Here's how the part is built. I have some questions about the finished solid (model axes, mm). Round coordinates to 2 decimals unless told otherwise and drop trailing zeros. Order: outer loops, then holes, each group sorted by start corner. A loop starts at its lowest first (then second) coordinate and runs counter-clockwise, first axis right, second up.
```python
from build123d import *

# Parameters (mm, degrees)
SKETCH1_W           = 20
SKETCH1_H           = 60
SKETCH1_R           = 3.3
BOSS_EXTRUDE1_DEPTH = 9.5
CHAMFER1_SIZE       = 0.3


with BuildPart() as part:
    # Sketch1 → Boss-Extrude1 (new body)
    with BuildSketch(Plane(origin=(0, 0, 0), x_dir=(1, 0, 0), z_dir=(0, 1, 0))):
        Rectangle(SKETCH1_W, SKETCH1_H)
        with Locations((0, 23)):
            Circle(SKETCH1_R, mode=Mode.SUBTRACT)
        with Locations((0, -23)):
            Circle(SKETCH1_R, mode=Mode.SUBTRACT)
    extrude(amount=BOSS_EXTRUDE1_DEPTH)

    # Chamfer1
    chamfer1_edges = [part.edges().sort_by_distance(p)[0] for p in [
        (-10, 4.75, -30),
        (10, 4.75, -30),
        (10, 4.75, 30),
        (-10, 4.75, 30),
    ]]
    chamfer(chamfer1_edges, length=CHAMFER1_SIZE)


solid = part.part
```
1. I need wall thicknesses on probe 1 along Z at (x, y) = (0, 4.5); probe 2 along X at (y, z) = (6.75, -23); probe 3 along Z at (x, y) = (-1.5, 3.5). Which ranges of each line are inside material? Lowest first, please.
Evaluation:
probe 1: z = -30 to -26.3, -19.7 to 19.7, 26.3 to 30
probe 2: x = -10 to -3.3, 3.3 to 10
probe 3: z = -30 to -25.94, -20.06 to 20.06, 25.94 to 30
2. If we section it at C-C, the plane y = 8.25: Write out the boundary of the cut face in (x, z).
Evaluation:
outline: (-10, -29.7) - (-9.7, -30) - (9.7, -30) - (10, -29.7) - (10, 29.7) - (9.7, 30) - (-9.7, 30) - (-10, 29.7) - close; hole circle Ø6.6 at (0, -23); hole circle Ø6.6 at (0, 23)
3. If we section it at D-D, the plane z = 24: Write out the boundary of the cut face in (x, y), and give its area (3 significant figures).
Evaluation:
outline: (-10, 0) - (-3.14, 0) - (-3.14, 9.5) - (-10, 9.5) - close; (3.14, 0) - (10, 0) - (10, 9.5) - (3.14, 9.5) - close
area: 130 mm2
4. I'm going to push a flat-ended pin straight in: P1, Ø8.5, axis at x = 0, z = -23, coming from the +Y side. Where does the tip first touch, or does it pass through?
Evaluation:
P1: stops at y = 9.5
5. If we section it at B-B, the plane z = -23: Write out the boundary of the cut face in (x, y), and give its area (3 significant figures).
Evaluation:
outline: (-10, 0) - (-3.3, 0) - (-3.3, 9.5) - (-10, 9.5) - close; (3.3, 0) - (10, 0) - (10, 9.5) - (3.3, 9.5) - close
area: 127 mm2
6. If we section it at A-A, the plane x = 0: Write out the boundary of the cut face in (y, z), and give its area (3 significant figures).
Evaluation:
outline: (0, -30) - (9.5, -30) - (9.5, -26.3) - (0, -26.3) - close; (0, -19.7) - (9.5, -19.7) - (9.5, 19.7) - (0, 19.7) - close; (0, 26.3) - (9.5, 26.3) - (9.5, 30) - (0, 30) - close
area: 445 mm2
